```python
from build123d import *

# Parameters (mm, degrees)
F0_W     = 15.24
F0_H     = 64.68872
F1_DEPTH = 1.27
F2_W     = 15.24
F2_H     = 24.6126
F3_DEPTH = 1.27
F4_W     = 15.24
F4_H     = 24.6126
F5_DEPTH = 1.27


with BuildPart() as f1:
    # F0 (on Front) → F1 (new body)
    with BuildSketch(Plane.XZ):
        with Locations((-0.545189, -1.028404)):
            Rectangle(F0_W, F0_H)
    extrude(amount=F1_DEPTH)

    # F2 (on face) → F3 (join)
    with BuildSketch(Plane.XY.offset(31.315956)):
        with Locations((-0.545189, -13.5763)):
            Rectangle(F2_W, F2_H)
    extrude(amount=-F3_DEPTH)

    # F4 (on face) → F5 (join)
    with BuildSketch(Plane(origin=(0, 0, -33.372764), x_dir=(1, 0, 0), z_dir=(0, 0, -1))):
        with Locations((-0.545189, 13.5763)):
            Rectangle(F4_W, F4_H)
    extrude(amount=-F5_DEPTH)


solid = f1.part
```
For this review, take the finished solid that the model builds, in its own axes (mm). A direction names the side the tool comes from. Round coordinates to 2 decimals unless told otherwise and drop trailing zeros. Write each loop counter-clockwise with the first axis right and the second up, starting at its lowest first coordinate (ties: lowest second). Pieces come first, ordered by that corner, then holes. Notation, with made-up numbers: (66, 22) - (125, 22) arc R19 cw to (125, 30) - close; hole circle Ø8 at (41.5, 45). An arc over 180 degrees is marked (long way). Put each result on its own line as item: value.
Q1. We need section B-B (x = 4). Give the boundary of the cut face in (y, z).
Solved:
outline: (-25.88, -33.37) - (0, -33.37) - (0, 31.32) - (-25.88, 31.32) - (-25.88, 30.05) - (-1.27, 30.05) - (-1.27, -32.1) - (-25.88, -32.1) - close
Q2. Wall thickness on probe 1 along Z at (x, y) = (1.75, -11.75); probe 2 along Y at (x, z) = (-1.75, 8.5): over which ranges is each line inside the solid? List them lowest first.
Solved:
probe 1: z = -33.37 to -32.1, 30.05 to 31.32
probe 2: y = -1.27 to 0
Q3. We need section A-A (y = -14.75). Give the boundary of the cut face in (x, z).
Solved:
outline: (-8.17, -33.37) - (7.07, -33.37) - (7.07, -32.1) - (-8.17, -32.1) - close; (-8.17, 30.05) - (7.07, 30.05) - (7.07, 31.32) - (-8.17, 31.32) - close
Q4. Insertion check: pin 1 Ø5 at (x, z) = (1.5, 0.5) entering from +Y; pin 2 Ø5 at (y, z) = (-4.5, -22.5) entering from +X; pin 3 Ø7.5 at (x, z) = (1.5, -12) entering from -Y. Each pin has a flat end and moves straight along its axis. Give the tip position at first contact, or say it passes through.
Solved:
pin 1: stops at y = 0
pin 2: passes through
pin 3: stops at y = -1.27
Q5. Machinability: for faces 1 (the face through (-1, -14, -32.103)), 2 (the face through (-1, -25.883, 31)), which of the approach directions +Z, -Z, +X, -X, +Y, -Y give a long, thin tool a straight path to every point of the face, cutting with its end or side? Answer none if there is none.
Solved:
face 1: +X, -X, -Y
face 2: +Z, -Z, +X, -X, -Y
Q6. We need section C-C (z = 6). Give the boundary of the cut face in (x, y).
Solved:
outline: (-8.17, -1.27) - (7.07, -1.27) - (7.07, 0) - (-8.17, 0) - close
